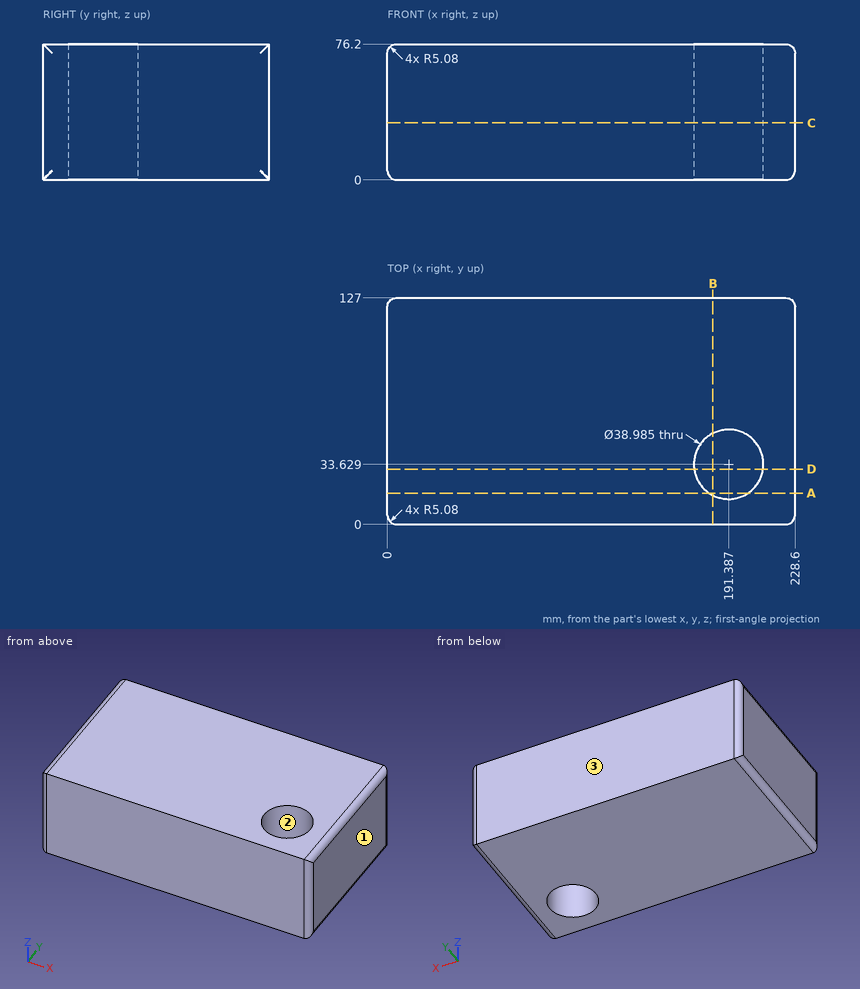
Can you work these out from the drawing? Everything is in mm from the part's minimum corner. Round coordinates to 2 decimals unless told otherwise and drop trailing zeros. Loops run counter-clockwise (first coordinate to the right, second up) from the corner with the lowest first, then second, coordinate; pieces in that order, holes last. Notation, with made-up numbers: (29.5, 25) - (72.5, 25) arc R8 ccw to (72.5, 39) - close; hole circle Ø11 at (13, 16.25). An arc over 180 degrees is marked (long way). One line per question, with ' | ' between items. Start each with the question number.
Q1. I want a section at B-B (x = 182.5). Write out the boundary of the cut face in (y, z), then the cut area to 3 significant figures.
Q2. I want a section at D-D (y = 31). Write out the boundary of the cut face in (x, z), then the cut area to 3 significant figures.
Q3. We'd pull the mould along Y, two halves only. Please class the marked faces 1, 2 and 3: +Y half, -Y half, draft (parallel to the pull), parting line (faces both ways), or undercut.
Q4. I want a section at C-C (z = 32). Write out the boundary of the cut face in (x, y) (1 decimal).
Q5. I want a section at A-A (y = 17.5). Write out the boundary of the cut face in (x, z), then the cut area to 3 significant figures.
Q6. Please list where these lines run through material, in increasing order: line 1 (X direction, y = 122, z = 48); line 2 (Y direction, x = 182, z = 24.5) (1 decimal); line 3 (Y direction, x = 208, z = 29.5) (1 decimal). Write a range as [from, to].
Response values:
1) outline: (0, 0) - (16.28, 0) - (16.28, 76.2) - (0, 76.2) - close; (50.98, 0) - (127, 0) - (127, 76.2) - (50.98, 76.2) - close | area: 7,030 mm²
2) outline: (0, 5.08) arc R5.08 ccw to (5.08, 0) - (172.07, 0) - (172.07, 76.2) - (5.08, 76.2) arc R5.08 ccw to (0, 71.12) - close; (210.7, 0) - (223.52, 0) arc R5.08 ccw to (228.6, 5.08) - (228.6, 71.12) arc R5.08 ccw to (223.52, 76.2) - (210.7, 76.2) - close | area: 14,500 mm²
3) face 1: draft | face 2: undercut | face 3: +Y half
4) outline: (0, 5.1) arc R5.1 ccw to (5.1, 0) - (223.5, 0) arc R5.1 ccw to (228.6, 5.1) - (228.6, 121.9) arc R5.1 ccw to (223.5, 127) - (5.1, 127) arc R5.1 ccw to (0, 121.9) - close; hole circle Ø39 at (191.4, 33.6)
5) outline: (0, 5.08) arc R5.08 ccw to (5.08, 0) - (180.44, 0) - (180.44, 76.2) - (5.08, 76.2) arc R5.08 ccw to (0, 71.12) - close; (202.33, 0) - (223.52, 0) arc R5.08 ccw to (228.6, 5.08) - (228.6, 71.12) arc R5.08 ccw to (223.52, 76.2) - (202.33, 76.2) - close | area: 15,700 mm²
6) line 1: x = [0, 228.6] | line 2: y = [0, 16.5], [50.7, 127] | line 3: y = [0, 23.4], [43.8, 127]
